from build123d import *

# Parameters (mm, degrees)
SKETCH1_R                = 6.35
BOSS_EXTRUDE1_DEPTH      = 304.8
SKETCH2_R                = 19.05
BOSS_EXTRUDE2_DEPTH      = 25.4
BOSS_EXTRUDE2_DEPTH_BACK = 25.4
CUT_EXTRUDE1_REACH       = 52.8
SKETCH3_R                = 6.35


with BuildPart() as part:
    # Sketch1 → Boss-Extrude1 (new body)
    with BuildSketch(Plane(origin=(0, 0, 0), x_dir=(0, 0, -1), z_dir=(1, 0, 0))):
        Circle(SKETCH1_R)
    extrude(amount=BOSS_EXTRUDE1_DEPTH)

    # Sketch2 → Boss-Extrude2 (add, two sides)
    with BuildSketch(Plane.XY) as boss_extrude2_sk:
        Circle(SKETCH2_R)
    extrude(amount=BOSS_EXTRUDE2_DEPTH)
    extrude(boss_extrude2_sk.sketch, amount=-BOSS_EXTRUDE2_DEPTH_BACK)

    # Sketch3 → Cut-Extrude1 (cut, up to next)
    with BuildSketch(Plane.XY.offset(25.4), mode=Mode.PRIVATE) as cut_extrude1_sk1:
        Circle(SKETCH3_R)
    cut_extrude1_tool1 = extrude(cut_extrude1_sk1.sketch, amount=-CUT_EXTRUDE1_REACH, mode=Mode.PRIVATE) & part.part
    add(cut_extrude1_tool1.solids().sort_by_distance((0, 0, 25.4))[0], mode=Mode.SUBTRACT)


solid = part.part
Read the model definition and answer for the solid it produces. Units are mm, in the model's axes. A direction names the side the tool comes from. Round coordinates to 2 decimals unless told otherwise and drop trailing zeros. Order: outer loops, then holes, each group sorted by start corner. A loop starts at its lowest first (then second) coordinate and runs counter-clockwise, first axis right, second up.
1) Flat-ended cylindrical pins translate along their axes: pin 1 (11.5 mm diameter, centred on x = 0, y = 0, fed in from +Z); pin 2 (3 mm diameter, centred on y = 12, z = -8, fed in from +X); pin 3 (8 mm diameter, centred on x = 14.5, z = 2.5, fed in from -Y). Find the tip coordinate at first contact, or state that the pin passes through.
2) The mould has two halves that part along X. Classify faces 3 (the face through (304.8, 0, 0)), 4 (the face through (-5, 5, -25.4)), 5 (the face through (-1.38, -6.2, 0.36)): released by +X, released by -X, zero draft, split by the parting line, or undercut.
3) The part is cut by section B-B on y = 0. Write down the section's boundary in (x, z).
4) The part is cut by section D-D on x = 188. Write down the section's boundary in (y, z).
5) The part is cut by section C-C on z = -11. Write down the section's boundary in (x, y), plus the area to 3 significant figures.
6) For faces 1 (the face through (-5, 5, 25.4)), 2 (the face through (159.37, -6.2, 1.38)), determine the directions among +Z, -Z, +X, -X, +Y, -Y from which every point of the face is accessible in a straight line to the end or side of a thin tool.
7) Straight lines are drawn through the part: L1, parallel to Y at x = 0, z = 5; L2, parallel to Y at x = 277.5, z = 0.5; L3, parallel to X at y = 4.5, z = 16. For each, find the intervals that lie inside material, in ascending order.
8) The part is cut by section A-A on x = 0. Write down the section's boundary in (y, z).
Resolved:
1. pin 1: passes through
1. pin 2: stops at x = 15.9
1. pin 3: stops at y = -15.9
2. face 3: released by +X
2. face 4: zero draft
2. face 5: undercut
3. outline: (-19.05, -25.4) - (-6.35, -25.4) - (-6.35, 25.4) - (-19.05, 25.4) - close; (6.35, -25.4) - (19.05, -25.4) - (19.05, -6.35) - (304.8, -6.35) - (304.8, 6.35) - (19.05, 6.35) - (19.05, 25.4) - (6.35, 25.4) - close
4. outline: circle Ø12.7 at (0, 0)
5. outline: circle Ø38.1 at (0, 0); hole circle Ø12.7 at (0, 0)
5. area: 1,010 mm2
6. face 1: +Z, +X, -X, +Y, -Y
6. face 2: +X
7. L1: y = -19.05 to -6.35, 6.35 to 19.05
7. L2: y = -6.33 to 6.33
7. L3: x = -18.51 to -4.48, 4.48 to 18.51
8. outline: (-19.05, -25.4) - (-6.35, -25.4) - (-6.35, 25.4) - (-19.05, 25.4) - close; (6.35, -25.4) - (19.05, -25.4) - (19.05, 25.4) - (6.35, 25.4) - close
